```python
from build123d import *

# Parameters (mm, degrees)
SKETCH102_R  = 5
PAD032_DEPTH = 12
FILLET001_R  = 4


with BuildPart() as part:
    # Sketch101 → Revolution001 (revolve)
    with BuildSketch(Plane.YZ):
        Polygon((-7.15, -9.5), (-9.5, -9.5), (-9.5, 37), (-17.75, 37), (-17.75, 47), (0, 47), (0, -21.8), (-7.15, -21.8), align=None)
    revolve(axis=Axis((0, 0, 0), (0, 0, 1)))

    # Sketch102 → Pad032 (new body, symmetric)
    with BuildSketch(Plane.XZ):
        Circle(SKETCH102_R)
    extrude(amount=PAD032_DEPTH, both=True)

    # Fillet001
    fillet001_edges = [part.edges().sort_by_distance(p)[0] for p in [
        (0, 9.5, 37),
    ]]
    fillet(fillet001_edges, radius=FILLET001_R)


solid = part.part
```
The listing builds one solid part. Answer for the finished solid, in the listing's coordinates (mm). A direction names the side the tool comes from. Coordinates: 2 decimals unless noted, no trailing zeros. Write each loop counter-clockwise with the first axis right and the second up, starting at its lowest first coordinate (ties: lowest second). Pieces come first, ordered by that corner, then holes. Notation, with made-up numbers: (68.5, -40) - (103.5, -40) arc R10 cw to (103.5, -21) - close; hole circle Ø1 at (-28, 79). An arc over 180 degrees is marked (long way). Return JSON: item names as keys, results as strings. Group by question number.
Q1. The part is cut by section D-D on z = 18. Write down the section's boundary in (x, y).
Q2. For a pull along Z with two mould halves and no side action, classify faces 4 (the flat face through (0, 0, -21.8)), 5 (the cylindrical face through (7.09, 0.93, -15.56)), 6 (the cylindrical face through (-0.651, -10.502, 4.957)) as +Z half, -Z half, draft (parallel to the pull), parting line (faces both ways), or undercut.
Q3. Find the intervals of material crossed by line 1 along Z through (x, y) = (-8, 14); line 2 along Z through (x, y) = (3, -7.5); line 3 along Y through (x, z) = (-5.5, -17.5), in increasing order. Write a range as [from, to].
Q4. Which of the six approach directions +Z, -Z, +X, -X, +Y, -Y give full straight-line access (tool end or side, diameter ignored) to faces 1 (the cylindrical face through (0.42, 9.49, 12.05)), 2 (the flat face through (6.4, -3.6, -9.5)), 3 (the flat face through (0, 12, 0))?
Q5. The part is cut by section C-C on x = 0. Write down the section's boundary in (y, z), and give its area (3 significant figures).
Q6. The part is cut by section B-B on z = 0. Write down the section's boundary in (x, y), and give its area (3 significant figures).
Q7. The part is cut by section A-A on y = 0. Write down the section's boundary in (x, z), and give its area (3 significant figures).
Q8. Flat-ended cylindrical pins translate along their axes: pin 1 Ø8 at (x, y) = (13.5, -7.5) entering from -Z; pin 2 Ø11 at (x, z) = (-0.5, 2.5) entering from -Y; pin 3 Ø5 at (x, z) = (-0.5, 2) entering from +Y. Find the tip coordinate at first contact, or state that the pin passes through.
Evaluation:
{
 "1": {"outline": "circle Ø19 at (0, 0)"},
 "2": {"face 4": "-Z half", "face 5": "draft", "face 6": "undercut"},
 "3": {"line 1": "z = [37, 47]", "line 2": "z = [-9.5, 47]", "line 3": "y = [-4.57, 4.57]"},
 "4": {"face 1": "none", "face 2": "-Z", "face 3": "-Z, +X, -X, +Y"},
 "5": {"outline": "(-17.75, 37) - (-13.5, 37) arc R4 cw to (-9.5, 33) - (-9.5, 5) - (-12, 5) - (-12, -5) - (-9.5, -5) - (-9.5, -9.5) - (-7.15, -9.5) - (-7.15, -21.8) - (7.15, -21.8) - (7.15, -9.5) - (9.5, -9.5) - (9.5, -5) - (12, -5) - (12, 5) - (9.5, 5) - (9.5, 33) arc R4 cw to (13.5, 37) - (17.75, 37) - (17.75, 47) - (-17.75, 47) - close", "area": "1,470 mm2"},
 "6": {"outline": "(-5, -12) - (5, -12) - (5, -8.08) arc R9.5 ccw to (5, 8.08) - (5, 12) - (-5, 12) - (-5, 8.08) arc R9.5 ccw to (-5, -8.08) - close", "area": "343 mm2"},
 "7": {"outline": "(-17.75, 37) - (-13.5, 37) arc R4 cw to (-9.5, 33) - (-9.5, -9.5) - (-7.15, -9.5) - (-7.15, -21.8) - (7.15, -21.8) - (7.15, -9.5) - (9.5, -9.5) - (9.5, 33) arc R4 cw to (13.5, 37) - (17.75, 37) - (17.75, 47) - (-17.75, 47) - close", "area": "1,420 mm2"},
 "8": {"pin 1": "stops at z = 36.43", "pin 2": "stops at y = -12", "pin 3": "stops at y = 12"}
}
